Check sheet for the modelled part. Datum: model origin and axes. Units: mm. A direction names the side the tool comes from. Round coordinates to 2 decimals unless told otherwise and drop trailing zeros. Order: outer loops, then holes, each group sorted by start corner. A loop starts at its lowest first (then second) coordinate and runs counter-clockwise, first axis right, second up.
Autodesk Inventor part; units mm, degrees
ref_plane "YZ Plane" through (0, 0, 0) normal (1, 0, 0) x (0, 1, 0)
ref_plane "XZ Plane" through (0, 0, 0) normal (0, 1, 0) x (-1, 0, 0)
ref_plane "XY Plane" through (0, 0, 0) normal (0, 0, 1) x (1, 0, 0)
sketch "Sketch1" plane through (0, 0, 0) normal (0, 0, 1) x (1, 0, 0)
  line L0 (19.05, -6.35) -> (-19.05, -6.35)
  line L1 (-19.05, -6.35) -> (-19.05, 6.35)
  line L2 (-19.05, 6.35) -> (19.05, 6.35)
  line L3 (19.05, 6.35) -> (19.05, -6.35)
  line L4 (19.05, -6.35) -> (-19.05, 6.35) construction
  line L5 (-19.05, -6.35) -> (19.05, 6.35) construction
  point P0 (0, 0)
  dimension "d0" = 38.1
  dimension "d1" = 12.7
extrude "Extrusion1" add sketch "Sketch1" along normal blind 12.7
sketch "Sketch2" plane through (-19.05, 6.35, 0) normal (0, 1, 0) x (1, 0, 0)
  line L0 (0, 0) -> (0, -12.7) construction
  line L1 (12.7, -6.35) -> (25.4, -6.35) construction
  line L2 (38.1, 0) -> (0, 0) construction
  line L3 (38.1, -12.7) -> (0, -12.7) construction
  point P0 (19.05, 0)
  point P1 (0, -6.35)
  point P2 (19.05, -6.35)
  point P3 (19.05, 0)
  point P4 (19.05, 0)
  dimension "d4" = 12.7
  dimension "d20" = 6.35
sketch "Sketch3" plane through (0, 0, 12.7) normal (0, 0, 1) x (1, 0, 0)
  line L0 (-12.7, 0) -> (12.7, 0) construction
  line L1 (-19.05, 6.35) -> (-19.05, -6.35) construction
  line L2 (19.05, 6.35) -> (-19.05, 6.35) construction
  point P0 (0, 0)
  point P1 (-19.05, 0)
  point P2 (0, 0)
  point P3 (0, 6.35)
  dimension "d12" = 25.4
hole "Hole2" at (-12.7, 0, 12.7) at (12.7, 0, 12.7) direction (0, 0, -1) diameter 5.1054 end through all
hole "Hole3" at (-6.35, 6.35, 6.35) at (6.35, 6.35, 6.35) direction (0, -1, 0) diameter 6.7564 depth 2.54 tip angle 118
fillet "Fillet1" radius 3.175 4 edges at (-19.05, 6.35, 6.35) (-19.05, -6.35, 6.35) (19.05, 6.35, 6.35) (19.05, -6.35, 6.35)
properties part number "CL7-GB-004" material "Aluminum 6061"
Item 1: Sectioned sample at A-A (x = -12.7). Record the cut outline in (y, z).
Answer:
outline: (-6.35, 0) - (-2.55, 0) - (-2.55, 12.7) - (-6.35, 12.7) - close; (2.55, 0) - (6.35, 0) - (6.35, 12.7) - (2.55, 12.7) - close
Item 2: Scan lines: line 1 along X through (y, z) = (0, 8.5); line 2 along Y through (x, z) = (12.7, 9); line 3 along X through (y, z) = (1.25, 12). Record each from-to range of solid material in increasing order.
Answer:
line 1: x = -19.05 to -15.25, -10.15 to 10.15, 15.25 to 19.05
line 2: y = -6.35 to -2.55, 2.55 to 6.35
line 3: x = -19.05 to -14.93, -10.47 to 10.47, 14.93 to 19.05
Item 3: Release check for a two-part mould opening along X. For faces 3 (the flat face through (19.05, 0, 6)), 4 (the flat face through (0, 0, 0)), 5 (the cylindrical face through (5.335, 5.062, 9.572)) record: released by +X, released by -X, zero draft, split by the parting line, or undercut.
Answer:
face 3: released by +X
face 4: zero draft
face 5: undercut
Item 4: Sectioned sample at B-B (y = 0). Record the cut outline in (x, z).
Answer:
outline: (-19.05, 0) - (-15.25, 0) - (-15.25, 12.7) - (-19.05, 12.7) - close; (-10.15, 0) - (10.15, 0) - (10.15, 12.7) - (-10.15, 12.7) - close; (15.25, 0) - (19.05, 0) - (19.05, 12.7) - (15.25, 12.7) - close
Item 5: Sectioned sample at C-C (z = 10.25). Record the cut outline in (x, y) (3 decimals).
Answer:
outline: (-19.05, -3.175) arc R3.175 ccw to (-15.875, -6.35) - (15.875, -6.35) arc R3.175 ccw to (19.05, -3.175) - (19.05, 3.175) arc R3.175 ccw to (15.875, 6.35) - (-15.875, 6.35) arc R3.175 ccw to (-19.05, 3.175) - close; hole circle Ø5.105 at (-12.7, 0); hole circle Ø5.105 at (12.7, 0)
Item 6: Go/stop test with a flat-tipped pin: P1, Ø4, axis at x = 6.35, z = 6.35, coming from the +Y side. Record where the tip stops, or that it passes through.
Answer:
P1: stops at y = 2.98
Item 7: Access from +Z, -Z, +X, -X, +Y, -Y to the whole of each face (thin tool, end or side, straight path). Record for faces 1 (the cylindrical face through (-7.365, 5.062, 9.572)), 2 (the cylindrical face through (15.192, 0.553, 6.261)).
Answer:
face 1: +Y
face 2: +Z, -Z
Item 8: Sectioned sample at D-D (y = -1.5). Record the cut outline in (x, z).
Answer:
outline: (-19.05, 0) - (-14.77, 0) - (-14.77, 12.7) - (-19.05, 12.7) - close; (-10.63, 0) - (10.63, 0) - (10.63, 12.7) - (-10.63, 12.7) - close; (14.77, 0) - (19.05, 0) - (19.05, 12.7) - (14.77, 12.7) - close
